```python
from build123d import *

# Parameters (mm, degrees)
SKETCH1_W                  = 80
SKETCH1_H                  = 80
BOSS_EXTRUDE1_DEPTH        = 8
CUT_EXTRUDE3_DEPTH         = 8
SKETCH5_R                  = 5.5
CUT_EXTRUDE4_DEPTH         = 8
F_4_0MM_DOWEL_HOLE1_D      = 4
F_4_0MM_DOWEL_HOLE1_DEPTH  = 2
F_4_0MM_DOWEL_HOLE2_REACH  = 115.42
F_4_0MM_DOWEL_HOLE2_BORE_R = 2
SKETCH11_W                 = 3
SKETCH11_H                 = 6
CUT_EXTRUDE5_DEPTH         = 8
CUT_EXTRUDE7_DEPTH         = 8
FILLET1_R                  = 4


with BuildPart() as part:
    # Sketch1 → Boss-Extrude1 (new body)
    with BuildSketch(Plane(origin=(0, 0, 0), x_dir=(0, 0, -1), z_dir=(1, 0, 0))):
        with Locations((-40, 40)):
            Rectangle(SKETCH1_W, SKETCH1_H)
    extrude(amount=BOSS_EXTRUDE1_DEPTH)

    # Sketch4 → Cut-Extrude3 (cut)
    with BuildSketch(Plane.ZY):
        Polygon((4.857641634, 41), (39, 76.795358795), (39, 41), align=None)
        Polygon((41.052631579, 76.897437673), (41.052631579, 41), (76.997364954, 41), align=None)
        Polygon((41.052631579, 39), (76.997364954, 39), (41.052631579, 3.102562327), align=None)
        Polygon((39, 39), (39, 3.204641205), (4.857641634, 39), align=None)
        Polygon((2, 7), (2, 0), (40, 0), (18.478318003, 22.654402102), align=None)
        Polygon((2, 9.758622845), (2, 38.05), (2.95, 39), (17.100819079, 24.10440097), align=None)
        Polygon((2, 41.95), (2, 70.241377155), (17.100819079, 55.89559903), (2.95, 41), align=None)
        Polygon((2, 80), (2, 73), (18.478318003, 57.345597898), (40, 80), align=None)
    extrude(amount=-CUT_EXTRUDE3_DEPTH, mode=Mode.SUBTRACT)

    # Sketch5 → Cut-Extrude4 (cut)
    with BuildSketch(Plane(origin=(8, 0, 0), x_dir=(0, 0, -1), z_dir=(1, 0, 0))):
        with Locations((-67, 70)):
            Circle(SKETCH5_R)
    extrude(amount=-CUT_EXTRUDE4_DEPTH, mode=Mode.SUBTRACT)

    # Ø4.0mm Dowel Hole1
    with Locations(Plane(origin=(0, 0, 0), x_dir=(-1, 0, 0), z_dir=(0, 0, -1))):
        with Locations((-3.917697329, 76), (-3.917697329, 4)):
            Hole(F_4_0MM_DOWEL_HOLE1_D / 2, depth=F_4_0MM_DOWEL_HOLE1_DEPTH)

    # Ø4.0mm Dowel Hole2 bore → Ø4.0mm Dowel Hole2 (cut, up to next)
    with BuildSketch(Plane.XY.offset(80), mode=Mode.PRIVATE) as f_4_0mm_dowel_hole2_sk1:
        with Locations((4.558585212, 70)):
            Circle(F_4_0MM_DOWEL_HOLE2_BORE_R)
    f_4_0mm_dowel_hole2_tool1 = extrude(f_4_0mm_dowel_hole2_sk1.sketch, amount=-F_4_0MM_DOWEL_HOLE2_REACH, mode=Mode.PRIVATE) & part.part
    add(f_4_0mm_dowel_hole2_tool1.solids().sort_by_distance((4.558585, 70, 80))[0], mode=Mode.SUBTRACT)

    # Sketch11 → Cut-Extrude5 (cut)
    with BuildSketch(Plane.ZY):
        with Locations((75.2, 70)):
            Rectangle(SKETCH11_W, SKETCH11_H)
    extrude(amount=-CUT_EXTRUDE5_DEPTH, mode=Mode.SUBTRACT)

    # Sketch15 → Cut-Extrude7 (cut)
    with BuildSketch(Plane.ZY):
        Polygon((43.882922576, 3.102562327), (76.997364954, 3.102562327), (76.997364954, 36.17343307), align=None)
    extrude(amount=-CUT_EXTRUDE7_DEPTH, mode=Mode.SUBTRACT)

    # Fillet1
    fillet1_edges = [part.edges().sort_by_distance(p)[0] for p in [
        (8, 0, 1),
        (0, 0, 1),
        (8, 80, 1),
        (0, 80, 1),
    ]]
    fillet(fillet1_edges, radius=FILLET1_R - 0.0001)  # a hair under: the kernel refuses the full size


solid = part.part
```
Could you check a few things on this model? Use its own coordinates, in mm. A direction names the side the tool comes from. Give positions to 0.01 mm unless a question says otherwise; leave off trailing zeros. Loops run counter-clockwise (first coordinate to the right, second up) from the corner with the lowest first, then second, coordinate; pieces in that order, holes last. Notation, with made-up numbers: (79.5, -1.75) -> (105.5, -1.75) arc R13 cw to (105.5, 4.25) -> close; hole circle Ø2 at (86.25, 56.5). An arc over 180 degrees is marked (long way). Put each result on its own line as item: value.
(1) Thinking about a two-plate mould opening in Z: for faces 5 (the face through (5, 78, 2)), 6 (the face through (4, 78, 1)), 7 (the face through (4, 39, 0)), which applies, pulls with the +Z half, pulls with the -Z half, needs draft (parallel to the pull), parting line crosses it, or undercut?
Computed:
face 5: undercut
face 6: needs draft
face 7: pulls with the -Z half
(2) Imagine slicing it at B-B on z = 67. Write out the boundary of the cut face in (x, y), plus the area to 3 significant figures.
Computed:
outline: (0, 0) -> (8, 0) -> (8, 3.1) -> (0, 3.1) -> close; (0, 26.19) -> (8, 26.19) -> (8, 29.02) -> (0, 29.02) -> close; (0, 39) -> (8, 39) -> (8, 41) -> (0, 41) -> close; (0, 50.98) -> (8, 50.98) -> (8, 64.5) -> (0, 64.5) -> close; (0, 75.5) -> (8, 75.5) -> (8, 80) -> (0, 80) -> close
area: 208 mm^2
(3) Imagine slicing it at C-C on z = 20. Write out the boundary of the cut face in (x, y), plus the area to 3 significant figures.
Computed:
outline: (0, 21.05) -> (8, 21.05) -> (8, 23.12) -> (0, 23.12) -> close; (0, 39) -> (8, 39) -> (8, 41) -> (0, 41) -> close; (0, 56.88) -> (8, 56.88) -> (8, 58.95) -> (0, 58.95) -> close
area: 49.2 mm^2
(4) I'm going to push flat-ended pins straight in: pin 1 Ø3 at (x, z) = (6.5, 26) entering from +Y; pin 2 Ø4 at (x, z) = (3, 63) entering from -Y; pin 3 Ø2.5 at (x, z) = (3, 22) entering from -Y; pin 4 Ø3 at (x, y) = (4.56, 70) entering from +Z. Where does each tip first touch, or does it pass through?
Computed:
pin 1: y = 66.84
pin 2: y = 0
pin 3: y = 17.63
pin 4: z = 61.71
(5) For faces 1 (the face through (2.971, 68.783, 72.923)), 2 (the face through (3.944, 68.514, 29.089)), 3 (the face through (6.859, 78.797, 0.986)), 4 (the face through (2, 70, 73.7)), which set-ups out of +Z, -Z, +X, -X, +Y, -Y let a thin tool reach every point of the face, with its end or its side?
Computed:
face 1: +Z
face 2: +X, -X, +Y
face 3: -Z, +X, +Y
face 4: +X, -X
(6) Please list where these lines run through material, in increasing order: probe 1 along Z at (x, y) = (5.25, 45.5) (3 decimals); probe 2 along Z at (x, y) = (4, 30); probe 3 along Y at (x, z) = (2.5, 62). Write a range as [from, to].
Computed:
probe 1: [0, 2], [7.225, 9.15], [39, 41.053], [72.491, 80]
probe 2: [0, 2], [11.5, 13.44], [39, 41.05], [67.99, 70.82], [77, 80]
probe 3: [0, 3.1], [21.2, 24.02], [39, 41], [55.98, 67.71], [72.29, 80]
(7) Imagine slicing it at A-A on y = 28. Write out the boundary of the cut face in (x, z).
Computed:
outline: (0, 0) -> (8, 0) -> (8, 2) -> (0, 2) -> close; (0, 13.4) -> (8, 13.4) -> (8, 15.35) -> (0, 15.35) -> close; (0, 39) -> (8, 39) -> (8, 41.05) -> (0, 41.05) -> close; (0, 65.98) -> (8, 65.98) -> (8, 68.81) -> (0, 68.81) -> close; (0, 77) -> (8, 77) -> (8, 80) -> (0, 80) -> close
(8) Imagine slicing it at D-D on y = 43. Write out the boundary of the cut face in (x, z).
Computed:
outline: (0, 0) -> (8, 0) -> (8, 2) -> (0, 2) -> close; (0, 4.85) -> (8, 4.85) -> (8, 6.77) -> (0, 6.77) -> close; (0, 39) -> (8, 39) -> (8, 41.05) -> (0, 41.05) -> close; (0, 74.99) -> (8, 74.99) -> (8, 80) -> (0, 80) -> close
